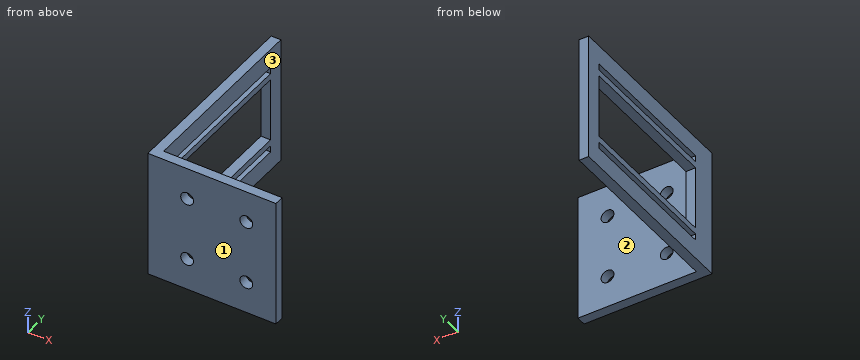
from build123d import *

# Parameters (mm, degrees)
BOSS_EXTRUDE1_DEPTH = 40
SKETCH2_R           = 2
CUT_EXTRUDE1_DEPTH  = 40
SKETCH3_W           = 2
SKETCH3_H           = 47
SKETCH3_W_2         = 20
CUT_EXTRUDE2_DEPTH  = 83.462112512


with BuildPart() as part:
    # Sketch1 → Boss-Extrude1 (new body)
    with BuildSketch(Plane.XY):
        Polygon((0, 0), (-40, 0), (-40, 60), (-37, 60), (-37, 3), (0, 3), align=None)
    extrude(amount=BOSS_EXTRUDE1_DEPTH)

    # Sketch2 → Cut-Extrude1 (cut)
    with BuildSketch(Plane(origin=(0, 3, 0), x_dir=(1, 0, 0), z_dir=(0, 1, 0))):
        with Locations(Location((-9.25, -30, 0), (0, 0, 270))):
            Circle(SKETCH2_R)
        with Locations(Location((-27.75, -30, 0), (0, 0, 270))):
            Circle(SKETCH2_R)
        with Locations(Location((-27.75, -10, 0), (0, 0, 270))):
            Circle(SKETCH2_R)
        with Locations(Location((-9.25, -10, 0), (0, 0, 270))):
            Circle(SKETCH2_R)
    extrude(amount=-CUT_EXTRUDE1_DEPTH, mode=Mode.SUBTRACT)

    # Sketch3 → Cut-Extrude2 (cut, through all)
    with BuildSketch(Plane.ZY.offset(40)):
        with Locations((33, 31.5)):
            Rectangle(SKETCH3_W, SKETCH3_H)
        with Locations((7, 31.5)):
            Rectangle(SKETCH3_W, SKETCH3_H)
        with Locations((20, 31.5)):
            Rectangle(SKETCH3_W_2, SKETCH3_H)
    extrude(amount=-CUT_EXTRUDE2_DEPTH, mode=Mode.SUBTRACT)


solid = part.part
CAD build for the part. Positions are in the model's coordinates, mm. Face numbers are marked on the shaded views. Round coordinates to 2 decimals unless told otherwise and drop trailing zeros. Loops run counter-clockwise (first coordinate to the right, second up) from the corner with the lowest first, then second, coordinate; pieces in that order, holes last. Notation, with made-up numbers: M 14.5,-33.5 L 31.5,-33.5 A26 ccw 31.5,-14.5 Z; hole C 66.5,-26.75 d4. An arc over 180 degrees is marked long. One line per question, with ' | ' between items. Start each with the question number.
Item 1: Cut at B-B, the plane x = -27.75. Write the cut outline in (y, z), plus the area to 3 significant figures.
Item 2: Wall check: line 1 (Z direction, x = -9, y = 2); line 2 (X direction, y = 1.05, z = 10); line 3 (Y direction, x = -10, z = 23.5). Give the ranges that are in metal, low to high.
Item 3: Cut at C-C, the plane y = 34. Write the cut outline in (x, z).
Item 4: Two-plate mould, pull along Y, no slides. Class the marked faces 1, 2 and 3: pulls with the +Y half, pulls with the -Y half, needs draft (parallel to the pull), parting line crosses it, or undercut.
Item 5: Pin check, flat tips, straight feed: pin 1 Ø1.5 at (x, y) = (-38.5, 25) entering from -Z; pin 2 Ø1 at (x, z) = (-11, 28) entering from +Y; pin 3 Ø6 at (y, z) = (38, 30) entering from +X. Stop position of each tip, or through.
Item 6: Cut at D-D, the plane z = 4. Write the cut outline in (x, y), plus the area to 3 significant figures.
Item 7: Cut at A-A, the plane z = 23.5. Write the cut outline in (x, y), plus the area to 3 significant figures.
Responses:
1) outline: M 0,0 L 3,0 L 3,8 L 0,8 Z; M 0,12 L 3,12 L 3,28 L 0,28 Z; M 0,32 L 3,32 L 3,40 L 0,40 Z | area: 96.0 mm²
2) line 1: z = 0 to 8.02, 11.98 to 28.02, 31.98 to 40 | line 2: x = -40 to -29.75, -25.75 to -11.25, -7.25 to 0 | line 3: y = 0 to 3
3) outline: M -40,0 L -37,0 L -37,6 L -40,6 Z; M -40,8 L -37,8 L -37,10 L -40,10 Z; M -40,30 L -37,30 L -37,32 L -40,32 Z; M -40,34 L -37,34 L -37,40 L -40,40 Z
4) face 1: pulls with the -Y half | face 2: pulls with the +Y half | face 3: needs draft
5) pin 1: stops at z = 0 | pin 2: stops at y = 3 | pin 3: stops at x = -37
6) outline: M -40,0 L 0,0 L 0,3 L -37,3 L -37,60 L -40,60 Z | area: 291 mm²
7) outline: M -40,0 L 0,0 L 0,3 L -37,3 L -37,8 L -40,8 Z; M -40,55 L -37,55 L -37,60 L -40,60 Z | area: 150 mm²
